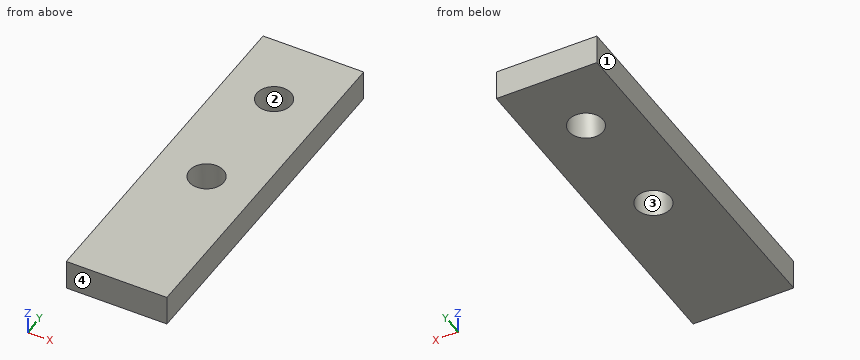
Autodesk Inventor part; units mm, degrees
ref_plane "YZ Plane" through (0, 0, 0) normal (1, 0, 0) x (0, 1, 0)
ref_plane "XZ Plane" through (0, 0, 0) normal (0, 1, 0) x (-1, 0, 0)
ref_plane "XY Plane" through (0, 0, 0) normal (0, 0, 1) x (1, 0, 0)
sketch "Sketch1" plane through (0, 0, 0) normal (0, 0, 1) x (1, 0, 0)
  line L0 (0, 0) -> (10, 0)
  line L1 (10, 0) -> (10, 35)
  line L2 (10, 35) -> (0, 35)
  line L3 (0, 35) -> (0, 0)
  dimension "d0" = 10
  dimension "d1" = 35
extrude "Extrusion1" add sketch "Sketch1" along normal blind 3
sketch "Sketch2" plane through (0, 0, 3) normal (0, 0, 1) x (1, 0, 0)
  line L0 (10, 35) -> (0, 35)
  line L1 (0, 35) -> (0, 0)
  point P0 (5, 28)
  point P1 (5, 16)
  dimension "d4" = 7
  dimension "d5" = 5
  dimension "d6" = 12
  dimension "d7" = 5
hole "Hole1" at (5, 28, 3) at (5, 16, 3) direction (0, 0, -1) diameter 3.4 end through all
sketch "Sketch3" plane through (0, 0, 3) normal (0, 0, 1) x (1, 0, 0)
  point P0 (0, 0)
sketch "Sketch4" plane through (0, 0, 3) normal (0, 0, 1) x (1, 0, 0)
  point P0 (0, 0)
properties part number "servoPipeConnection"
Model file for the job. Use its own axes, mm. Face numbers are marked on the shaded views. Give positions to 0.01 mm unless a question says otherwise; leave off trailing zeros. Loops run counter-clockwise (first coordinate to the right, second up) from the corner with the lowest first, then second, coordinate; pieces in that order, holes last. Notation, with made-up numbers: (-0.75, 3.5) - (41.25, 3.5) arc R33 cw to (41.25, 35.5) - close; hole circle Ø11 at (35, 9.5). An arc over 180 degrees is marked (long way). One line per item, written item: value. Start each with the question number.
1. Probe L1, parallel to Y at x = 5, z = 1.25; L2, parallel to X at y = 28, z = 2.45; L3, parallel to Y at x = 6.25, z = 1. List the from-to ranges inside material, lowest first. Write a range as from..to.
2. Pin check, flat tip, straight feed: pin 1 (5.5 mm diameter, centred on x = 5, y = 16, fed in from +Z). Stop position of the tip, or through.
3. Slice it at A-A (y = 28). List the corners of the cut face in (x, z).
4. Pull direction X, two halves, no side cores. Call the marked faces 1, 2, 3 and 4: pulls with the +X half, pulls with the -X half, needs draft (parallel to the pull), parting line crosses it, or undercut.
5. Slice it at C-C (z = 2.6). List the corners of the cut face in (x, y), plus the area to 3 significant figures.
6. Slice it at B-B (x = 5). List the corners of the cut face in (y, z), plus the area to 3 significant figures.
Solution:
1. L1: y = 0..14.3, 17.7..26.3, 29.7..35
1. L2: x = 0..3.3, 6.7..10
1. L3: y = 0..14.85, 17.15..26.85, 29.15..35
2. pin 1: stops at z = 3
3. outline: (0, 0) - (3.3, 0) - (3.3, 3) - (0, 3) - close; (6.7, 0) - (10, 0) - (10, 3) - (6.7, 3) - close
4. face 1: pulls with the -X half
4. face 2: undercut
4. face 3: undercut
4. face 4: needs draft
5. outline: (0, 0) - (10, 0) - (10, 35) - (0, 35) - close; hole circle Ø3.4 at (5, 16); hole circle Ø3.4 at (5, 28)
5. area: 332 mm^2
6. outline: (0, 0) - (14.3, 0) - (14.3, 3) - (0, 3) - close; (17.7, 0) - (26.3, 0) - (26.3, 3) - (17.7, 3) - close; (29.7, 0) - (35, 0) - (35, 3) - (29.7, 3) - close
6. area: 84.6 mm^2
